from build123d import *

# Parameters (mm, degrees)
F1_DEPTH = 535
F2_R     = 3.4
F3_DEPTH = 30
F4_R     = 3.4
F5_DEPTH = 30


with BuildPart() as f1:
    # F0 (on Front) → F1 (new body)
    with BuildSketch(Plane.XZ):
        Polygon((0, 50), (0, 0), (60, 0), (60, 50), (57, 50), (42, 35), (42, 29), (30, 29), (18, 29), (18, 35), (3, 50), align=None)
    extrude(amount=F1_DEPTH)

    # F2 (on face) → F3 (cut)
    with BuildSketch(Plane(origin=(0, 0, 0), x_dir=(1, 0, 0), z_dir=(0, 0, -1))):
        with Locations((30, 520)):
            Circle(F2_R)
        with Locations((30, 505)):
            Circle(F2_R)
        with Locations((30, 490)):
            Circle(F2_R)
        with Locations((30, 45)):
            Circle(F2_R)
        with Locations((30, 30)):
            Circle(F2_R)
        with Locations((30, 15)):
            Circle(F2_R)
    extrude(amount=-F3_DEPTH, mode=Mode.SUBTRACT)

    # F4 (on face) → F5 (cut)
    with BuildSketch(Plane(origin=(0, 0, 0), x_dir=(0, -1, 0), z_dir=(-1, 0, 0))):
        with Locations((30, 9)):
            Circle(F4_R)
        with Locations((505, 9)):
            Circle(F4_R)
    extrude(amount=-F5_DEPTH, mode=Mode.SUBTRACT)


solid = f1.part
Geometry check sheet. Reference: the model listing, model coordinates, mm. A direction names the side the tool comes from. Coordinates: 2 decimals unless noted, no trailing zeros. Order: outer loops, then holes, each group sorted by start corner. A loop starts at its lowest first (then second) coordinate and runs counter-clockwise, first axis right, second up. Notation, with made-up numbers: (32, 31.5) - (69, 31.5) arc R12 cw to (69, 43.5) - close; hole circle Ø8 at (6.25, 87). An arc over 180 degrees is marked (long way). One line per item, written item: value.
(1) Sectioned sample at C-C (x = 51). Enter the section's corners in (y, z), and give its area (3 significant figures).
Data:
outline: (-535, 0) - (0, 0) - (0, 44) - (-535, 44) - close
area: 23,500 mm^2
(2) Release check for a two-part mould opening along X. For faces 3 (the face through (30, -535, 20)), 4 (the face through (11, -264, 42)), 5 (the face through (60, -264, 25)), 6 (the face through (0, -264, 25)) record: +X half, -X half, draft (parallel to the pull), parting line (faces both ways), or undercut.
Data:
face 3: draft
face 4: undercut
face 5: +X half
face 6: -X half
(3) Access from +Z, -Z, +X, -X, +Y, -Y to the whole of each face (thin tool, end or side, straight path). Record for faces 1 (the face through (30, -264, 0)), 2 (the face through (30, -264, 29)).
Data:
face 1: -Z, +X, -X, +Y, -Y
face 2: +Z, +Y, -Y
(4) Sectioned sample at A-A (z = 44). Enter the section's corners in (x, y).
Data:
outline: (0, -535) - (9, -535) - (9, 0) - (0, 0) - close; (51, -535) - (60, -535) - (60, 0) - (51, 0) - close
(5) Thickness scan on probe 1 along X at (y, z) = (-30, 23); probe 2 along X at (y, z) = (-342.5, 30.5); probe 3 along Z at (x, y) = (26, -120.5). Record the ranges inside material, lowest first. Write a range as from..to.
Data:
probe 1: x = 0..26.6, 33.4..60
probe 2: x = 0..18, 42..60
probe 3: z = 0..29
(6) Sectioned sample at B-B (y = -96.5). Enter the section's corners in (x, z).
Data:
outline: (0, 0) - (60, 0) - (60, 50) - (57, 50) - (42, 35) - (42, 29) - (18, 29) - (18, 35) - (3, 50) - (0, 50) - close
(7) Depth check by flat-ended pin: pin 1 Ø10 at (x, y) = (43.5, -354) entering from +Z; pin 2 Ø5.5 at (y, z) = (-30, 9) entering from -X; pin 3 Ø4 at (y, z) = (-505, 9) entering from -X. Enter the tip coordinate at first touch or a pass-through.
Data:
pin 1: stops at z = 41.5
pin 2: stops at x = 32
pin 3: stops at x = 32.75
